Part model, mm, in its own coordinate system. Face numbers are marked on the shaded views. A direction names the side the tool comes from. Round coordinates to 2 decimals unless told otherwise and drop trailing zeros. Write each loop counter-clockwise with the first axis right and the second up, starting at its lowest first coordinate (ties: lowest second). Pieces come first, ordered by that corner, then holes. Notation, with made-up numbers: (-11, 75) -> (32, 75) arc R4 ccw to (32, 80) -> close; hole circle Ø3 at (58, 45). An arc over 180 degrees is marked (long way). Use CSV: the item, a comma, the result in double quotes. Start each with the question number.
(1) Saw through at B-B (z = 18). Give the cut face in (x, y).
(2) Probe line 1 (X direction, y = 19.5, z = 15); line 2 (Z direction, x = 0, y = 25.85); line 3 (Y direction, x = -3, z = 14.5). List the from-to ranges inside material, lowest first. Write a range as [from, to].
(3) Two-plate mould, pull along X, no slides. Class the marked faces 4, 5 and 6: released by +X, released by -X, zero draft, split by the parting line, or undercut.
(4) Saw through at A-A (x = 0). Give the cut face in (y, z), plus the area to 3 significant figures.
(5) Saw through at C-C (y = 22.5). Give the cut face in (x, z), plus the area to 3 significant figures.
(6) Saw through at D-D (y = 28). Give the cut face in (x, z), plus the area to 3 significant figures.
(7) Drop flat-ended pins along their axis: pin 1 (2 mm diameter, centred on y = 32, z = 18.5, fed in from -X); pin 2 (1.1 mm diameter, centred on x = 0.5, y = 26, fed in from -Z); pin 3 (1.8 mm diameter, centred on y = 30, z = 15, fed in from +X); pin 4 (3.5 mm diameter, centred on x = 0, y = 11, fed in from +Z). Give the stop position or say it passes through.
(8) Which spindle directions (+Z, -Z, +X, -X, +Y, -Y) get a long thin tool onto all of the face, cutting with end or side? Do the marked faces 1, 2 and 3. Say none if no direction does.
```python
from build123d import *

# Parameters (mm, degrees)
PAD011_DEPTH    = 14.6
SKETCH023_W     = 12
SKETCH023_H     = 10
PAD012_DEPTH    = 1
FILLET003_R     = 0.5
SKETCH024_R     = 0.455689
PAD013_DEPTH    = 7.5
SKETCH025_W     = 12
SKETCH025_H     = 10
PAD014_DEPTH    = 1
SKETCH026_R     = 1.9
POCKET008_DEPTH = 7.5
SKETCH027_R     = 1.45
PAD015_DEPTH    = 9
FILLET004_R     = 0.5
POCKET009_DEPTH = 10


with BuildPart() as part:
    # Sketch022 → Pad011 (new body)
    with BuildSketch(Plane.XZ):
        with BuildLine():
            Line((-3.5, 19.873397), (3.5, 19.873397))
            ThreePointArc((3.117362, 9.873397), (5.995612, 14.770585), (3.5, 19.873397))
            Line((3.117362, 9.873397), (-3.117362, 9.873397))
            ThreePointArc((-3.5, 19.873397), (-5.995612, 14.770585), (-3.117362, 9.873397))
        make_face()
    extrude(amount=PAD011_DEPTH)

    # Sketch023 (on Face5 of Pad011) → Pad012 (join)
    with BuildSketch(Plane(origin=(0, 0, 0), x_dir=(1, 0, 0), z_dir=(0, 1, 0))):
        with Locations((0, -15)):
            Rectangle(SKETCH023_W, SKETCH023_H)
    extrude(amount=PAD012_DEPTH)

    # Fillet003
    fillet003_edges = [part.edges().sort_by_distance(p)[0] for p in [
        (6, 0.5, 20),
        (6, 0.5, 10),
        (-6, 0.5, 10),
        (-6, 0.5, 20),
    ]]
    fillet(fillet003_edges, radius=FILLET003_R)

    # Sketch024 → Pad013 (join)
    with BuildSketch(Plane.XZ):
        with Locations((-5.376898, 19.295448)):
            Circle(SKETCH024_R)
        with Locations((-5.395437, 10.616136)):
            Circle(SKETCH024_R)
        with Locations((5.395437, 10.616136)):
            Circle(SKETCH024_R)
        with Locations((5.376898, 19.295448)):
            Circle(SKETCH024_R)
    extrude(amount=-PAD013_DEPTH)

    # Sketch025 → Pad014 (join)
    with BuildSketch(Plane.XZ.offset(-7.5)):
        with Locations((0, 15)):
            Rectangle(SKETCH025_W, SKETCH025_H)
    extrude(amount=PAD014_DEPTH)

    # Sketch026 (on Face32 of Pad014) → Pocket008 (cut)
    with BuildSketch(Plane(origin=(0, 7.5, 0), x_dir=(1, 0, 0), z_dir=(0, 1, 0))):
        with Locations((0, -15)):
            Circle(SKETCH026_R)
    extrude(amount=-POCKET008_DEPTH, mode=Mode.SUBTRACT)

    # Sketch027 (on Face35 of Pocket008) → Pad015 (join, symmetric)
    with BuildSketch(Plane(origin=(0, 7.5, 0), x_dir=(1, 0, 0), z_dir=(0, 1, 0))):
        with Locations((0, -15)):
            Circle(SKETCH027_R)
    extrude(amount=PAD015_DEPTH, both=True)

    # Fillet004
    fillet004_edges = [part.edges().sort_by_distance(p)[0] for p in [
        (-6, 7, 20),
        (-6, 7, 10),
        (6, 7, 10),
        (6, 7, 20),
    ]]
    fillet(fillet004_edges, radius=FILLET004_R)

    # Sketch028 → Pocket009 (cut)
    with BuildSketch(Plane.XZ.offset(-7)):
        with BuildLine():
            ThreePointArc((0.9, 13.863118), (1.45, 15), (0.9, 16.136882))
            Line((0.9, 13.863118), (0.9, 16.136882))
        make_face()
    extrude(amount=-POCKET009_DEPTH, mode=Mode.SUBTRACT)


with BuildPart() as part_1:
    # Body007 placement: moved
    add(part.part.moved(Location((0, 19, 0))))


solid = part_1.part
```
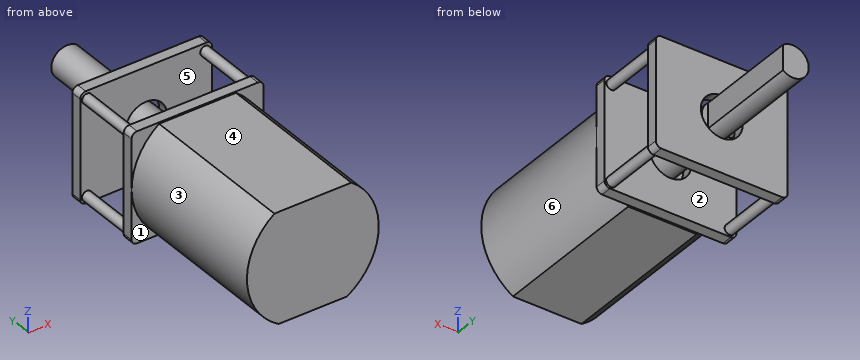
Answers:
1,outline,"(-6, 19) -> (-5.2, 19) -> (-5.2, 4.4) -> (5.2, 4.4) -> (5.2, 19) -> (6, 19) -> (6, 20) -> (-6, 20) -> close; (-6, 25.5) -> (6, 25.5) -> (6, 26.5) -> (-6, 26.5) -> close"
2,line 1,"x = [-6, -1.9], [-1.45, 1.45], [1.9, 6]"
2,line 2,"z = [10, 13.1], [13.55, 16.45], [16.9, 20]"
2,line 3,"y = [4.4, 20], [25.5, 26.5]"
3,face 4,"zero draft"
3,face 5,"undercut"
3,face 6,"released by +X"
4,outline,"(4.4, 9.87) -> (19, 9.87) -> (19, 10) -> (20, 10) -> (20, 13.1) -> (19, 13.1) -> (19, 13.55) -> (35.5, 13.55) -> (35.5, 16.45) -> (19, 16.45) -> (19, 16.9) -> (20, 16.9) -> (20, 20) -> (19, 20) -> (19, 19.87) -> (4.4, 19.87) -> close; (25.5, 10) -> (26.5, 10) -> (26.5, 13.1) -> (25.5, 13.1) -> close; (25.5, 16.9) -> (26.5, 16.9) -> (26.5, 20) -> (25.5, 20) -> close"
4,area,"206 mm²"
5,outline,"circle Ø0.91 at (-5.4, 10.62); circle Ø0.91 at (-5.38, 19.3); circle Ø2.9 at (0, 15); circle Ø0.91 at (5.38, 19.3); circle Ø0.91 at (5.4, 10.62)"
5,area,"9.21 mm²"
6,outline,"(0.9, 13.86) -> (0.9, 16.14) arc R1.45 ccw (long way) to start"
6,area,"5.73 mm²"
7,pin 1,"passes through"
7,pin 2,"stops at z = 10"
7,pin 3,"stops at x = 0.9"
7,pin 4,"stops at z = 19.87"
8,face 1,"-Y"
8,face 2,"none"
8,face 3,"-X, -Y"
